Geometry check sheet. Reference: the model listing, model coordinates, mm. A direction names the side the tool comes from. Give positions to 0.01 mm unless a question says otherwise; leave off trailing zeros. Loops run counter-clockwise (first coordinate to the right, second up) from the corner with the lowest first, then second, coordinate; pieces in that order, holes last. Notation, with made-up numbers: (-35.75, -13) - (-28.75, -13) arc R8 ccw to (-28.75, -4) - close; hole circle Ø2 at (27, 4). An arc over 180 degrees is marked (long way). Use a Markdown table: item, result. Add a question column.
1. Set-up check for faces 5 (the flat face through (-20, -2, 1)), 6 (the cylindrical face through (20.065, 1.774, 0.493)): record each of +Z, -Z, +X, -X, +Y, -Y from which the full face is reachable in a straight line by a thin tool's end or side.
2. Cross-section at C-C on x = 0. Enter the section's corners in (y, z) (3 decimals), and give its area (3 significant figures).
3. Material ranges on L1, parallel to Y at x = -22, z = 1.4; L2, parallel to Y at x = -22, z = 0.55 (3 decimals); L3, parallel to X at y = -22, z = 0.3 (3 decimals), recorded low to high.
4. Draft check along Y on faces 1 (the cylindrical face through (-3, 0.1, 1.5)), 2 (the flat face through (42.5, -1, 1)), 3 (the cylindrical face through (2.5, 0.8, 0.5)), 4 (the flat face through (-1, 42.5, 1)). Enter one of: pulls with the +Y half, pulls with the -Y half, needs draft (parallel to the pull), parting line crosses it, or undercut.
5. Cross-section at D-D on y = 22. Enter the section's corners in (x, z) (3 decimals), and give its area (4 significant figures).
6. Cross-section at A-A on x = 22. Enter the section's corners in (y, z) (3 decimals), and give its area (3 significant figures).
from build123d import *

# Parameters (mm, degrees)
SKETCH_W     = 85
SKETCH_H     = 85
SKETCH_R     = 2.625
PAD_DEPTH    = 2
SKETCH001_R  = 3
POCKET_DEPTH = 1


with BuildPart() as part:
    # Sketch → Pad (new body)
    with BuildSketch(Plane.XY):
        Rectangle(SKETCH_W, SKETCH_H)
        with Locations((-22, 22)):
            Circle(SKETCH_R, mode=Mode.SUBTRACT)
        with Locations((-22, 0)):
            Circle(SKETCH_R, mode=Mode.SUBTRACT)
        with Locations((-22, -22)):
            Circle(SKETCH_R, mode=Mode.SUBTRACT)
        Circle(SKETCH_R, mode=Mode.SUBTRACT)
        with Locations((22, 22)):
            Circle(SKETCH_R, mode=Mode.SUBTRACT)
        with Locations((22, 0)):
            Circle(SKETCH_R, mode=Mode.SUBTRACT)
        with Locations((22, -22)):
            Circle(SKETCH_R, mode=Mode.SUBTRACT)
    extrude(amount=PAD_DEPTH)

    # Sketch001 (on Face13 of Pad) → Pocket (cut)
    with BuildSketch(Plane.XY.offset(2)):
        with Locations((-22, 22)):
            Circle(SKETCH001_R)
        with Locations((-22, 0)):
            Circle(SKETCH001_R)
        with Locations((-22, -22)):
            Circle(SKETCH001_R)
        Circle(SKETCH001_R)
        with Locations((22, 0)):
            Circle(SKETCH001_R)
        with Locations((22, 22)):
            Circle(SKETCH001_R)
        with Locations((22, -22)):
            Circle(SKETCH001_R)
    extrude(amount=-POCKET_DEPTH, mode=Mode.SUBTRACT)


solid = part.part
Values found:
| question | item | result |
|---|---|---|
| 1 | face 5 | +Z |
| 1 | face 6 | +Z, -Z |
| 2 | outline | (-42.5, 0) - (-2.625, 0) - (-2.625, 1) - (-3, 1) - (-3, 2) - (-42.5, 2) - close; (2.625, 0) - (42.5, 0) - (42.5, 2) - (3, 2) - (3, 1) - (2.625, 1) - close |
| 2 | area | 159 mm2 |
| 3 | L1 | y = -42.5 to -25, -19 to -3, 3 to 19, 25 to 42.5 |
| 3 | L2 | y = -42.5 to -24.625, -19.375 to -2.625, 2.625 to 19.375, 24.625 to 42.5 |
| 3 | L3 | x = -42.5 to -24.625, -19.375 to 19.375, 24.625 to 42.5 |
| 4 | face 1 | undercut |
| 4 | face 2 | needs draft |
| 4 | face 3 | undercut |
| 4 | face 4 | pulls with the +Y half |
| 5 | outline | (-42.5, 0) - (-24.625, 0) - (-24.625, 1) - (-25, 1) - (-25, 2) - (-42.5, 2) - close; (-19.375, 0) - (19.375, 0) - (19.375, 1) - (19, 1) - (19, 2) - (-19, 2) - (-19, 1) - (-19.375, 1) - close; (24.625, 0) - (42.5, 0) - (42.5, 2) - (25, 2) - (25, 1) - (24.625, 1) - close |
| 5 | area | 147.5 mm2 |
| 6 | outline | (-42.5, 0) - (-24.625, 0) - (-24.625, 1) - (-25, 1) - (-25, 2) - (-42.5, 2) - close; (-19.375, 0) - (-2.625, 0) - (-2.625, 1) - (-3, 1) - (-3, 2) - (-19, 2) - (-19, 1) - (-19.375, 1) - close; (2.625, 0) - (19.375, 0) - (19.375, 1) - (19, 1) - (19, 2) - (3, 2) - (3, 1) - (2.625, 1) - close; (24.625, 0) - (42.5, 0) - (42.5, 2) - (25, 2) - (25, 1) - (24.625, 1) - close |
| 6 | area | 136 mm2 |
